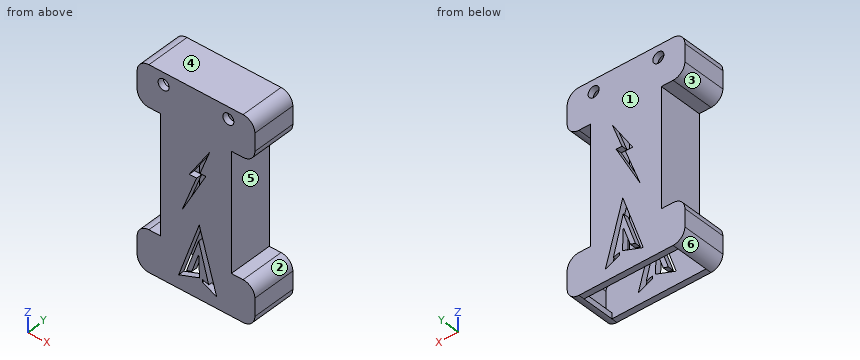
```python
from build123d import *

# Parameters (mm, degrees)
F0_W     = 30.48
F0_H     = 50.8
F1_DEPTH = 19.05
F2_R     = 5.08
F4_T     = -2.54
F3_R     = 2.3749
F5_DEPTH = 45.59299
F7_DEPTH = 16.68371
F8_DEPTH = 25.4


# Not quite as in the source:
# - a shell that OpenCascade refuses in one call is made with other operations: the cavity is built on its own and cut out


with BuildPart() as f1:
    # F0 (on Front) → F1 (new body)
    with BuildSketch(Plane.XZ):
        with Locations((-8.951122936, -13.8477537125)):
            Rectangle(F0_W, F0_H)
        Polygon((6.288877064, -39.2477537125), (-24.191122936, -39.2477537125), (-34.351122936, -39.2477537125), (-34.351122936, -57.0277537125), (16.448877064, -57.0277537125), (16.448877064, -39.2477537125), align=None)
        Polygon((16.448877064, 29.3322462875), (-34.351122936, 29.3322462875), (-34.351122936, 11.5522462875), (-24.191122936, 11.5522462875), (6.288877064, 11.5522462875), (16.448877064, 11.5522462875), align=None)
    extrude(amount=F1_DEPTH)

    # F2
    f2_edges = [f1.edges().sort_by_distance(p)[0] for p in [
        (-34.351123, -9.525, 11.552246),
        (16.448877, -9.525, 11.552246),
        (16.448877, -9.525, 29.332246),
        (-34.351123, -9.525, 29.332246),
        (-34.351123, -9.525, -39.247754),
        (-34.351123, -9.525, -57.027754),
        (16.448877, -9.525, -57.027754),
        (16.448877, -9.525, -39.247754),
    ]]
    fillet(f2_edges, radius=F2_R)

    # F4: a shell. OpenCascade refuses it in one call, so the cavity is built on its own and cut out:
    # the body offset inwards by the wall thickness, plus a prism from it out through each open face.
    f4_core = offset(f1.part, amount=F4_T, kind=Kind.INTERSECTION, mode=Mode.PRIVATE)
    f4_exits = [f4_core.faces().sort_by_distance(p)[0] for p in [
        (-8.951123, -9.525, -54.487754),
    ]]
    add(f4_core, mode=Mode.SUBTRACT)
    extrude(f4_exits, amount=-F4_T, mode=Mode.SUBTRACT)

    # F3 (on face) → F5 (cut)
    with BuildSketch(Plane.XZ.offset(19.05)):
        with Locations((-22.921122936, 24.2522462875)):
            Circle(F3_R)
        with Locations((5.018877064, 24.2522462875)):
            Circle(F3_R)
    extrude(amount=-F5_DEPTH, mode=Mode.SUBTRACT)

    # F6 (on face) → F7 (cut)
    with BuildSketch(Plane.XZ.offset(19.05)):
        Polygon((-7.217857521, -4.5538423583), (-3.042159602, 6.352733355), (-11.8417982012, -7.2901686653), (-8.6815273389, -7.2901686653), (-15.0396805257, -23.8231290132), (-4.6957456507, -4.5538423583), align=None)
    extrude(amount=-F7_DEPTH, mode=Mode.SUBTRACT)

    # F6 (on face) → F8 (cut)
    with BuildSketch(Plane.XZ.offset(19.05)):
        Polygon((-7.217857521, -4.5538423583), (-3.042159602, 6.352733355), (-11.8417982012, -7.2901686653), (-8.6815273389, -7.2901686653), (-15.0396805257, -23.8231290132), (-4.6957456507, -4.5538423583), align=None)
        Polygon((-7.5618713163, -26.2167993933), (-16.4136328948, -51.3810502087), (-7.4369557778, -48.071410507), (-7.7901184559, -38.5827049613), (-10.809615066, -47.1666878623), (-13.0202344465, -47.8591975347), (-7.7901184559, -32.9299127667), (-3.4719579703, -49.0020355231), (-6.1175874434, -48.071410507), (-6.1175874434, -49.2577214361), (0, -52.201025188), align=None)
    extrude(amount=-F8_DEPTH, mode=Mode.SUBTRACT)


solid = f1.part
```
Here's how the part is built. I have some questions about the finished solid (model axes, mm). Face numbers are marked on the shaded views. A direction names the side the tool comes from. Round coordinates to 2 decimals unless told otherwise and drop trailing zeros. Loops run counter-clockwise (first coordinate to the right, second up) from the corner with the lowest first, then second, coordinate; pieces in that order, holes last.
1. For the marked faces 1, 2 and 3, which set-ups out of +Z, -Z, +X, -X, +Y, -Y let a thin tool reach every point of the face, with its end or its side?
Answers:
face 1: +Z, -Z, +X, -X, +Y
face 2: +X, +Y, -Y
face 3: -X, +Y, -Y
2. Suppose I cut it at D-D, the plane z = -12.5. Please give me the cut outline in (x, y), and give its area (3 significant figures).
Answers:
outline: (-24.19, -19.05) - (-10.69, -19.05) - (-10.69, -16.51) - (-21.65, -16.51) - (-21.65, -2.54) - (-10.69, -2.54) - (-10.69, 0) - (-24.19, 0) - close; (-8.96, -19.05) - (6.29, -19.05) - (6.29, 0) - (-8.96, 0) - (-8.96, -2.54) - (3.75, -2.54) - (3.75, -16.51) - (-8.96, -16.51) - close
area: 217 mm2
3. If I drill on probe 1 along Z at (x, y) = (-29, -4.25); probe 2 along Y at (x, z) = (-6.5, 21.5); probe 3 along X at (y, z) = (-2.75, -25), over which ranges is the centre line in solid material (lowest first)?
Answers:
probe 1: z = -41.79 to -39.25, 11.55 to 14.09, 26.79 to 29.33
probe 2: y = -19.05 to -16.51, -2.54 to 0
probe 3: x = -24.19 to -21.65, 3.75 to 6.29
4. Will these pins go through, and if not, where does the flat tip stop? pin 1 (1 mm diameter, centred on x = -5.5, y = -8, fed in from -Z); pin 2 (4 mm diameter, centred on x = 5.02, z = 24.25, fed in from -Y); pin 3 (7 mm diameter, centred on y = -9.5, z = -14.5, fed in from +X); pin 4 (9.5 mm diameter, centred on y = -12.5, z = -21, fed in from -X).
Answers:
pin 1: stops at z = 26.79
pin 2: passes through
pin 3: stops at x = 6.29
pin 4: stops at x = -24.19
5. Suppose I cut it at C-C, the plane x = 1. Please give me the cut outline in (y, z), and give its area (3 significant figures).
Answers:
outline: (-19.05, -57.03) - (-16.51, -57.03) - (-16.51, 26.79) - (-2.54, 26.79) - (-2.54, -57.03) - (0, -57.03) - (0, 29.33) - (-19.05, 29.33) - close
area: 474 mm2
6. Thinking about a two-plate mould opening in Z: for the marked faces 4, 5 and 6, which applies, released by +Z, released by -Z, zero draft, split by the parting line, or undercut?
Answers:
face 4: released by +Z
face 5: undercut
face 6: released by -Z
7. Suppose I cut it at B-B, the plane z = 9. Please give me the cut outline in (x, y).
Answers:
outline: (-24.19, -19.05) - (6.29, -19.05) - (6.29, 0) - (-24.19, 0) - close; hole (-21.65, -16.51) - (3.75, -16.51) - (3.75, -2.54) - (-21.65, -2.54) - close
8. Suppose I cut it at A-A, the plane x = -27. Please give me the cut outline in (y, z).
Answers:
outline: (-19.05, -57.03) - (-16.51, -57.03) - (-16.51, -41.79) - (-2.54, -41.79) - (-2.54, -57.03) - (0, -57.03) - (0, -39.25) - (-19.05, -39.25) - close; (-19.05, 11.55) - (0, 11.55) - (0, 29.33) - (-19.05, 29.33) - close; hole (-16.51, 14.09) - (-2.54, 14.09) - (-2.54, 26.79) - (-16.51, 26.79) - close
